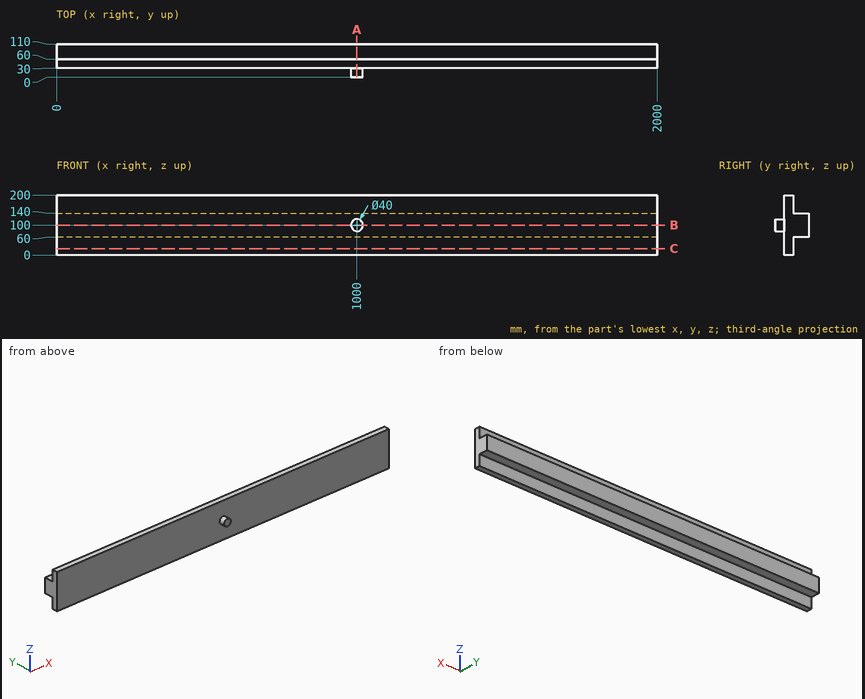
Verification items for this drawing (mm, ordinates from the low corner). Round coordinates to 2 decimals unless told otherwise and drop trailing zeros. Write each loop counter-clockwise with the first axis right and the second up, starting at its lowest first coordinate (ties: lowest second). Pieces come first, ordered by that corner, then holes. Notation, with made-up numbers: (-19.75, 33) - (27.25, 33) arc R11 cw to (27.25, 48) - close; hole circle Ø3 at (-36, 87.5). An arc over 180 degrees is marked (long way). Answer as a JSON object with one key per item and string values. Group by question number.
Q1. Thickness scan on line 1 (Y direction, x = 675.5, z = 158.5); line 2 (Y direction, x = 1448.5, z = 106.5); line 3 (Z direction, x = 1883, y = 71). Record the ranges inside material, lowest first.
Q2. Section check B-B, the plane z = 100. Enter the section's corners in (x, y).
Q3. Section check A-A, the plane x = 1000. Enter the section's corners in (y, z), plus the area to 3 significant figures.
Q4. Section check C-C, the plane z = 21.5. Enter the section's corners in (x, y).
Q5. Go/stop test with flat-tipped pins: pin 1 Ø6 at (x, z) = (334.5, 134.5) entering from -Y; pin 2 Ø2 at (y, z) = (20.5, 95) entering from +X; pin 3 Ø10 at (x, z) = (244, 27) entering from +Y. Record where each tip stops, or that it passes through.
Found:
{
 "1": {"line 1": "y = 30 to 60", "line 2": "y = 30 to 110", "line 3": "z = 60 to 140"},
 "2": {"outline": "(0, 30) - (980, 30) - (980, 0) - (1020, 0) - (1020, 30) - (2000, 30) - (2000, 110) - (0, 110) - close"},
 "3": {"outline": "(0, 80) - (30, 80) - (30, 0) - (60, 0) - (60, 60) - (110, 60) - (110, 140) - (60, 140) - (60, 200) - (30, 200) - (30, 120) - (0, 120) - close", "area": "11,200 mm^2"},
 "4": {"outline": "(0, 30) - (2000, 30) - (2000, 60) - (0, 60) - close"},
 "5": {"pin 1": "stops at y = 30", "pin 2": "stops at x = 1019.6", "pin 3": "stops at y = 60"}
}
